Could you check a few things on this model? Use its own coordinates, in mm. A direction names the side the tool comes from. Round coordinates to 2 decimals unless told otherwise and drop trailing zeros. Order: outer loops, then holes, each group sorted by start corner. A loop starts at its lowest first (then second) coordinate and runs counter-clockwise, first axis right, second up. Notation, with made-up numbers: (79, -9.75) - (109, -9.75) arc R18 ccw to (109, 0.25) - close; hole circle Ø11 at (-1.5, -5). An arc over 180 degrees is marked (long way). Return JSON: item names as keys, results as strings. Group by question number.
from build123d import *

# Parameters (mm, degrees)
SKETCH1_W           = 23.6
SKETCH1_H           = 53
BOSS_EXTRUDE2_DEPTH = 7.1
SHELL1_T            = -1.6
FILLET2_R           = 3
SKETCH7_W           = 12.2
SKETCH7_H           = 1.6
CUT_EXTRUDE1_DEPTH  = 3.1
SKETCH8_W           = 13.4
SKETCH8_H           = 1.6
CUT_EXTRUDE2_DEPTH  = 3.7
SKETCH9_W           = 3.55
SKETCH9_H           = 1
BOSS_EXTRUDE3_DEPTH = 3.2
SKETCH10_R          = 1.4
BOSS_EXTRUDE4_DEPTH = 7.1
SKETCH11_R          = 0.6
CUT_EXTRUDE4_DEPTH  = 7.1
FILLET3_R           = 1


with BuildPart() as part:
    # Sketch1 → Boss-Extrude2 (new body)
    with BuildSketch(Plane.XY):
        with Locations((-28.818351302, -28.026390465)):
            Rectangle(SKETCH1_W, SKETCH1_H)
    extrude(amount=BOSS_EXTRUDE2_DEPTH)

    # Shell1
    shell1_openings = [part.faces().sort_by_distance(p)[0] for p in [
        (-28.818351302, -28.026390465, 7.1),
    ]]
    offset(amount=SHELL1_T, openings=shell1_openings, kind=Kind.INTERSECTION)

    # Fillet2
    fillet2_edges = [part.edges().sort_by_distance(p)[0] for p in [
        (-40.618351302, -1.526390465, 3.55),
        (-17.018351302, -1.526390465, 3.55),
        (-17.018351302, -54.526390465, 3.55),
        (-40.618351302, -54.526390465, 3.55),
    ]]
    fillet(fillet2_edges, radius=FILLET2_R)

    # Sketch7 → Cut-Extrude1 (cut)
    with BuildSketch(Plane.XY.offset(7.1)):
        with Locations((-28.818351302, -53.726390465)):
            Rectangle(SKETCH7_W, SKETCH7_H)
    extrude(amount=-CUT_EXTRUDE1_DEPTH, mode=Mode.SUBTRACT)

    # Sketch8 → Cut-Extrude2 (cut)
    with BuildSketch(Plane.XY.offset(7.1)):
        with Locations((-28.818351302, -2.326390465)):
            Rectangle(SKETCH8_W, SKETCH8_H)
    extrude(amount=-CUT_EXTRUDE2_DEPTH, mode=Mode.SUBTRACT)

    # Sketch9 → Boss-Extrude3 (add)
    with BuildSketch(Plane.XY.offset(1.6)):
        with Locations((-20.393351302, -14.826390465)):
            Rectangle(SKETCH9_W, SKETCH9_H)
        with Locations((-37.243351302, -14.826390465)):
            Rectangle(SKETCH9_W, SKETCH9_H)
    extrude(amount=BOSS_EXTRUDE3_DEPTH)

    # Sketch10 → Boss-Extrude4 (add)
    with BuildSketch(Plane.XY.offset(7.1)):
        with Locations((-38.618351302, -52.426390465)):
            Circle(SKETCH10_R)
        with Locations((-19.018351302, -52.426390465)):
            Circle(SKETCH10_R)
        with Locations((-38.618351302, -27.126390465)):
            Circle(SKETCH10_R)
        with Locations((-19.018351302, -27.126390465)):
            Circle(SKETCH10_R)
        with Locations((-18.818351302, -3.626390465)):
            Circle(SKETCH10_R)
        with Locations((-38.618351302, -3.626390465)):
            Circle(SKETCH10_R)
    extrude(amount=-BOSS_EXTRUDE4_DEPTH)

    # Sketch11 → Cut-Extrude4 (cut)
    with BuildSketch(Plane.XY.offset(7.1)):
        with Locations((-38.618351302, -3.626390465)):
            Circle(SKETCH11_R)
        with Locations((-19.018351302, -3.626390465)):
            Circle(SKETCH11_R)
        with Locations((-38.618351302, -52.426390465)):
            Circle(SKETCH11_R)
        with Locations((-19.018351302, -52.426390465)):
            Circle(SKETCH11_R)
        with Locations((-38.618351302, -27.126390465)):
            Circle(SKETCH11_R)
        with Locations((-19.018351302, -27.126390465)):
            Circle(SKETCH11_R)
    extrude(amount=-CUT_EXTRUDE4_DEPTH, mode=Mode.SUBTRACT)

    # Fillet3
    fillet3_edges = [part.edges().sort_by_distance(p)[0] for p in [
        (-28.818351302, -1.526390465, 0),
        (-40.618351302, -28.026390465, 0),
        (-17.018351302, -28.026390465, 0),
        (-28.818351302, -54.526390465, 0),
        (-39.739671646, -2.405070122, 0),
        (-39.739671646, -53.647710809, 0),
        (-17.897030959, -53.647710809, 0),
        (-17.897030959, -2.405070122, 0),
    ]]
    fillet(fillet3_edges, radius=FILLET3_R)


solid = part.part
1) We'd pull the mould along X, two halves only. Please class faces 1 (the flat face through (-35.468, -15, 3)), 2 (the flat face through (-29, -54.526, 3)), 3 (the cylindrical face through (-17.9, -2.4, 4.1)): +X half, -X half, draft (parallel to the pull), parting line (faces both ways), or undercut.
2) For faces 4 (the cylindrical face through (-28.94, -54.24, 0.3)), 5 (the flat face through (-34.918, -54, 6)), 6 (the flat face through (-20, -15, 4.8)), which set-ups out of +Z, -Z, +X, -X, +Y, -Y let a thin tool reach every point of the face, with its end or its side?
3) I want a section at B-B, the plane y = -11. List the corners of the cut face in (x, z) for me.
4) Will these pins go through, and if not, where does the flat tip stop? pin 1 (2 mm diameter, centred on x = -26, y = -36, fed in from +Z); pin 2 (1.3 mm diameter, centred on x = -29, y = -2, fed in from +Z); pin 3 (1.9 mm diameter, centred on x = -19.02, y = -3.63, fed in from +Z); pin 4 (0.5 mm diameter, centred on y = -2.5, z = 6, fed in from -X).
5) I want a section at C-C, the plane x = -31.25. List the corners of the cut face in (y, z) for me.
6) If I drill on line 1 along X through (y, z) = (-12, 2.75); line 2 along Y through (x, z) = (-19.25, 1.25); line 3 along Y through (x, z) = (-27.25, 2), over which ranges is the centre line in solid material (lowest first)? Write a range as from..to.
7) I want a section at A-A, the plane z = 6.25. Give the number of separate pieces and of enclosed holes in the cut face, plus the area to 3 significant figures.
Outcome:
{
 "1": {"face 1": "undercut", "face 2": "draft", "face 3": "+X half"},
 "2": {"face 4": "-Z, +X, -X, -Y", "face 5": "+Z, +Y, -Y", "face 6": "+Z"},
 "3": {"outline": "(-40.62, 1) arc R1 ccw to (-39.62, 0) - (-18.02, 0) arc R1 ccw to (-17.02, 1) - (-17.02, 7.1) - (-18.62, 7.1) - (-18.62, 1.6) - (-39.02, 1.6) - (-39.02, 7.1) - (-40.62, 7.1) - close"},
 "4": {"pin 1": "z = 1.6", "pin 2": "z = 3.4", "pin 3": "z = 7.1", "pin 4": "x = -40.04"},
 "5": {"outline": "(-54.53, 1) arc R1 ccw to (-53.53, 0) - (-2.53, 0) arc R1 ccw to (-1.53, 1) - (-1.53, 3.4) - (-3.13, 3.4) - (-3.13, 1.6) - (-52.93, 1.6) - (-52.93, 4) - (-54.53, 4) - close"},
 "6": {"line 1": "-40.62..-39.02, -18.62..-17.02", "line 2": "-54.43..-52.98, -51.87..-27.68, -26.57..-4.18, -3.07..-1.63", "line 3": "-54.53..-52.93, -3.13..-1.53"},
 "7": {"separate pieces": "2", "enclosed holes": "6", "area": "199 mm^2"}
}
